For this review, take the finished solid that the model builds, in its own axes (mm). Face numbers are marked on the shaded views. A direction names the side the tool comes from. Give positions to 0.01 mm unless a question says otherwise; leave off trailing zeros. Write each loop counter-clockwise with the first axis right and the second up, starting at its lowest first coordinate (ties: lowest second). Pieces come first, ordered by that corner, then holes. Notation, with made-up numbers: (-27.75, 57.5) -> (-12.75, 57.5) arc R22 cw to (-12.75, 79.5) -> close; hole circle Ø10 at (17, 33). An arc over 180 degrees is marked (long way). Return JSON: item names as keys, results as strings.
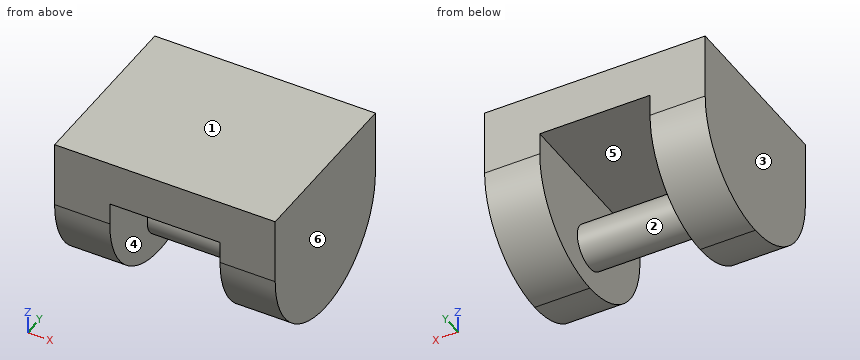
from build123d import *

# Parameters (mm, degrees)
SKETCH_1_W          = 10
SKETCH_1_H          = 8
EXTRUDE_1_DEPTH     = 3
EXTRUDE_2_DEPTH     = 10
SKETCH_4_W          = 5
SKETCH_4_H          = 8
CUT_EXTRUDE_1_DEPTH = 10
SKETCH_5_R          = 1
EXTRUDE_3_DEPTH     = 10
SKETCH_7_W          = 5
SKETCH_7_H          = 1
CUT_EXTRUDE_2_DEPTH = 10


with BuildPart() as part:
    # 草图1 → 凸台-拉伸1 (new body)
    with BuildSketch(Plane.XY):
        Rectangle(SKETCH_1_W, SKETCH_1_H)
    extrude(amount=EXTRUDE_1_DEPTH)

    # 草图3 → 凸台-拉伸2 (add)
    with BuildSketch(Plane(origin=(5, 0, 0), x_dir=(0, 0, -1), z_dir=(1, 0, 0))):
        with BuildLine():
            ThreePointArc((4, 0), (2.828427125, 2.828427125), (0, 4))
            Line((0, 4), (0, -4))
            ThreePointArc((0, -4), (2.828427125, -2.828427125), (4, 0))
        make_face()
    extrude(amount=-EXTRUDE_2_DEPTH)

    # 草图4 → 切除-拉伸1 (cut)
    with BuildSketch(Plane.XY):
        Rectangle(SKETCH_4_W, SKETCH_4_H)
    extrude(amount=-CUT_EXTRUDE_1_DEPTH, mode=Mode.SUBTRACT)

    # 草图5 → 凸台-拉伸3 (add)
    with BuildSketch(Plane.ZY.offset(5)):
        with Locations((-2, 0)):
            Circle(SKETCH_5_R)
    extrude(amount=-EXTRUDE_3_DEPTH)

    # 草图7 → 切除-拉伸2 (cut)
    with BuildSketch(Plane(origin=(0, -4, 0), x_dir=(-1, 0, 0), z_dir=(0, -1, 0))):
        with Locations((0, -0.5)):
            Rectangle(SKETCH_7_W, SKETCH_7_H)
    extrude(amount=-CUT_EXTRUDE_2_DEPTH, mode=Mode.SUBTRACT)


solid = part.part
1. For the marked faces 4, 5 and 6, list the 3-axis set-ups (+Z, -Z, +X, -X, +Y, -Y) from which the entire face can be reached by the end or side of a thin tool; tool diameter is ignored.
Results found:
{"face 4": "none", "face 5": "+Y, -Y", "face 6": "+Z, -Z, +X, +Y, -Y"}
2. The part is to be moulded in two halves that separate along Z. For the marked faces 1, 2 and 3, say which applies: +Z half, -Z half, draft (parallel to the pull), parting line (faces both ways), or undercut.
Results found:
{"face 1": "+Z half", "face 2": "undercut", "face 3": "draft"}
3. Add section D-D, the plane x = -3. State the section outline as (y, z) points, plus the area to 3 significant figures.
Results found:
{"outline": "(-4, 0) arc R4 ccw to (4, 0) -> (4, 3) -> (-4, 3) -> close", "area": "49.1 mm²"}
4. Add section A-A, the plane z = 0.75. State the section outline as (x, y) points, plus the area to 3 significant figures.
Results found:
{"outline": "(-5, -4) -> (-2.5, -4) -> (-2.5, 4) -> (-5, 4) -> close; (2.5, -4) -> (5, -4) -> (5, 4) -> (2.5, 4) -> close", "area": "40.0 mm²"}
5. Add section B-B, the plane x = 2.25. State the section outline as (y, z) points, plus the area to 3 significant figures.
Results found:
{"outline": "(-4, 1) -> (4, 1) -> (4, 3) -> (-4, 3) -> close; circle Ø2 at (0, -2)", "area": "19.1 mm²"}
6. Add section C-C, the plane y = -0.5. State the section outline as (x, z) points.
Results found:
{"outline": "(-5, -3.97) -> (-2.5, -3.97) -> (-2.5, -2.87) -> (2.5, -2.87) -> (2.5, -3.97) -> (5, -3.97) -> (5, 3) -> (-5, 3) -> close; hole (-2.5, -1.13) -> (2.5, -1.13) -> (2.5, 1) -> (-2.5, 1) -> close"}
7. To check wall thickness, follow probe 1 along X at (y, z) = (1.5, -1.5); probe 2 along Z at (x, y) = (-0.5, 1.75); probe 3 along Y at (x, z) = (1.75, -2). State the ranges of each line that lie inside material, in increasing order.
Results found:
{"probe 1": "x = -5 to -2.5, 2.5 to 5", "probe 2": "z = 1 to 3", "probe 3": "y = -1 to 1"}
8. For pin 1 (1.5 mm diameter, centred on x = 1, y = -1.5, fed in from -Z); pin 2 (1 mm diameter, centred on x = 0.5, y = -2, fed in from -Z), all flat-tipped, find the tip position at first contact; note any pin that passes through.
Results found:
{"pin 1": "stops at z = -2.66", "pin 2": "stops at z = 1"}
